Geometry: final body of the model. Coordinates: model frame, mm. A direction names the side the tool comes from. Round coordinates to 2 decimals unless told otherwise and drop trailing zeros. Loops run counter-clockwise (first coordinate to the right, second up) from the corner with the lowest first, then second, coordinate; pieces in that order, holes last. Notation, with made-up numbers: (76, 52.5) - (106, 52.5) arc R16 cw to (106, 58.5) - close; hole circle Ø6 at (-32.75, 78). An arc over 180 degrees is marked (long way). Answer as a JSON object with one key per item and string values. Group by question number.
Item 1: Line query: line 1 (Y direction, x = 0, z = -0.3); line 2 (X direction, y = -1.5, z = 0.3); line 3 (Y direction, x = 112.5, z = 0). Output: solid intervals per line, ascending.
Item 2: Section B-B (z = -0.25). Return the cut outline in (x, y), plus the area to 3 significant figures.
Item 3: Reachability of faces 4 (the face through (58, 5, 0)), 5 (the face through (60, -5, 0)), 6 (the face through (56, 0, 1.5)), 7 (the face through (10, 0, 0)) from +Z, -Z, +X, -X, +Y, -Y: full face, straight path, thin tool, end or side. Return the list, or none.
Item 4: Section A-A (x = 0). Return the cut outline in (y, z), plus the area to 3 significant figures.
Item 5: Draft query along Y for faces 1 (the face through (-7.496, -0.253, 0.021)), 2 (the face through (12, 1, 0)), 3 (the face through (56, 0, -1.5)). Return one class per face: released by +Y, released by -Y, zero draft, split by the parting line, or undercut.
Item 6: Section C-C (x = 64.5). Return the cut outline in (y, z).
Item 7: First-contact query: pin 1 (0.9 mm diameter, centred on x = 47.5, z = 0.5, fed in from +Y); pin 2 (1.5 mm diameter, centred on y = 4.5, z = 0, fed in from -X). Flat tips, straight axial feed; report the tip coordinate or a pass-through.
```python
from build123d import *

# Parameters (mm, degrees)
SKETCH_1_R      = 2
SKETCH_1_R_2    = 4
EXTRUDE_1_DEPTH = 1.5


with BuildPart() as part:
    # 草图1 → 凸台-拉伸1 (new, symmetric)
    with BuildSketch(Plane.XY):
        with BuildLine():
            Line((5.590169944, 5), (112.5, 5))
            ThreePointArc((112.5, 5), (117.5, 0), (112.5, -5))
            Line((112.5, -5), (5.590169944, -5))
            ThreePointArc((5.590169944, -5), (-7.5, 0), (5.590169944, 5))
        make_face()
        with Locations((112.5, 0)):
            Circle(SKETCH_1_R, mode=Mode.SUBTRACT)
        Circle(SKETCH_1_R_2, mode=Mode.SUBTRACT)
        with BuildLine():
            Line((11, 1), (14, 1))
            ThreePointArc((14, 1), (15, 0), (14, -1))
            Line((14, -1), (11, -1))
            ThreePointArc((11, -1), (10, 0), (11, 1))
        make_face(mode=Mode.SUBTRACT)
    extrude(amount=EXTRUDE_1_DEPTH, both=True)


solid = part.part
```
Values:
{
 "1": {"line 1": "y = -7.5 to -4, 4 to 7.5", "line 2": "x = -7.35 to -3.71, 3.71 to 111.18, 113.82 to 117.27", "line 3": "y = -5 to -2, 2 to 5"},
 "2": {"outline": "(5.59, -5) - (112.5, -5) arc R5 ccw to (112.5, 5) - (5.59, 5) arc R7.5 ccw (long way) to start; hole circle Ø8 at (0, 0); hole (11, -1) - (14, -1) arc R1 ccw to (14, 1) - (11, 1) arc R1 ccw to start; hole circle Ø4 at (112.5, 0)", "area": "1,200 mm^2"},
 "3": {"face 4": "+Z, -Z, +X, +Y", "face 5": "+Z, -Z, +X, -Y", "face 6": "+Z, +X, -X, +Y, -Y", "face 7": "+Z, -Z"},
 "4": {"outline": "(-7.5, -1.5) - (-4, -1.5) - (-4, 1.5) - (-7.5, 1.5) - close; (4, -1.5) - (7.5, -1.5) - (7.5, 1.5) - (4, 1.5) - close", "area": "21.0 mm^2"},
 "5": {"face 1": "split by the parting line", "face 2": "undercut", "face 3": "zero draft"},
 "6": {"outline": "(-5, -1.5) - (5, -1.5) - (5, 1.5) - (-5, 1.5) - close"},
 "7": {"pin 1": "stops at y = 5", "pin 2": "stops at x = -6.5"}
}
